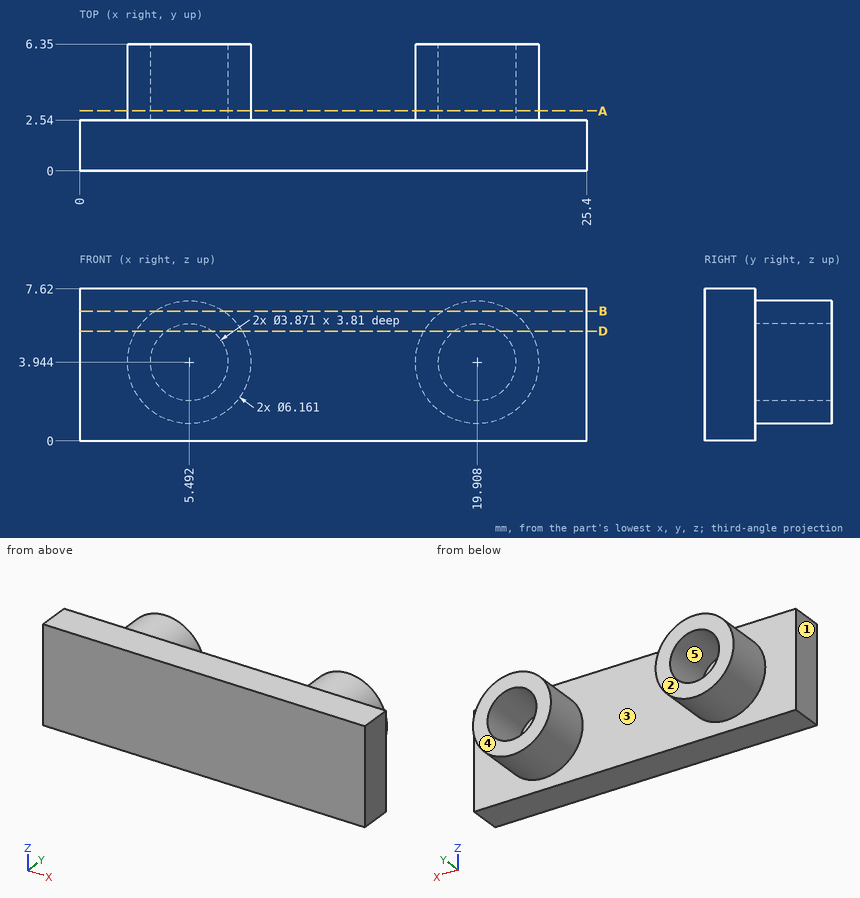
Study the drawing (mm; zero at the part's minimum x, y, z) and answer. A direction names the side the tool comes from. Give positions to 0.01 mm unless a question says otherwise; leave off trailing zeros. Loops run counter-clockwise (first coordinate to the right, second up) from the corner with the lowest first, then second, coordinate; pieces in that order, holes last. Notation, with made-up numbers: M 54.5,69 L 85.5,69 A31 ccw 85.5,103 Z; hole C -31,69.5 d10. An arc over 180 degrees is marked long. One line per item, written item: value. Start each with the question number.
1. Find section A-A (y = 3). Give the vertices of the cut face in (x, z) (1 decimal).
2. Find section B-B (z = 6.5). Give the vertices of the cut face in (x, y).
3. Determine the mould class of the marked faces 1, 2 and 3 for opening direction X: released by +X, released by -X, zero draft, split by the parting line, or undercut.
4. Each of these flat-tipped pins is pushed along its axis until it touches: P1, Ø4.5, axis at x = 20, z = 3.5, coming from the +Y side; P2, Ø3.5, axis at x = 19.91, z = 3.94, coming from the +Y side. Where does it stop, or does it pass through?
5. Find section D-D (z = 5.5). Give the vertices of the cut face in (x, y).
6. Find the intervals of material crossed by probe 1 along X at (y, z) = (4, 4); probe 2 along X at (y, z) = (3, 5.25) (1 decimal); probe 3 along X at (y, z) = (6.25, 1.5) (1 decimal), in increasing order.
7. Which of the six approach directions +Z, -Z, +X, -X, +Y, -Y give full straight-line access (tool end or side, diameter ignored) to the marked faces 4 and 5?
Reported:
1. outline: C 5.5,3.9 d6.2; C 19.9,3.9 d6.2; hole C 5.5,3.9 d3.9; hole C 19.9,3.9 d3.9
2. outline: M 0,0 L 25.4,0 L 25.4,2.54 L 21.63,2.54 L 21.63,6.35 L 18.19,6.35 L 18.19,2.54 L 7.21,2.54 L 7.21,6.35 L 3.77,6.35 L 3.77,2.54 L 0,2.54 Z
3. face 1: released by -X
3. face 2: zero draft
3. face 3: undercut
4. P1: stops at y = 6.35
4. P2: stops at y = 2.54
5. outline: M 0,0 L 25.4,0 L 25.4,2.54 L 22.57,2.54 L 22.57,6.35 L 21.06,6.35 L 21.06,2.54 L 18.76,2.54 L 18.76,6.35 L 17.25,6.35 L 17.25,2.54 L 8.15,2.54 L 8.15,6.35 L 6.64,6.35 L 6.64,2.54 L 4.34,2.54 L 4.34,6.35 L 2.83,6.35 L 2.83,2.54 L 0,2.54 Z
6. probe 1: x = 2.41 to 3.56, 7.43 to 8.57, 16.83 to 17.97, 21.84 to 22.99
6. probe 2: x = 2.7 to 4.1, 6.9 to 8.3, 17.1 to 18.5, 21.3 to 22.7
6. probe 3: x = 3.6 to 7.4, 18 to 21.8
7. face 4: +Z, -Z, +X, -X, +Y
7. face 5: +Y
